Input: part model. Units: mm. Frame: model coordinates. Face numbers are marked on the shaded views. A direction names the side the tool comes from. Coordinates: 2 decimals unless noted, no trailing zeros. Loops run counter-clockwise (first coordinate to the right, second up) from the corner with the lowest first, then second, coordinate; pieces in that order, holes last. Notation, with made-up numbers: (29, 38.5) -> (67, 38.5) arc R33 ccw to (67, 76.5) -> close; hole circle Ø5 at (-6, 40). An arc over 180 degrees is marked (long way). Answer as a JSON object with one key per item and string values.
Autodesk Inventor part; units mm, degrees
ref_plane "YZ Plane" through (0, 0, 0) normal (1, 0, 0) x (0, 1, 0)
ref_plane "XZ Plane" through (0, 0, 0) normal (0, 1, 0) x (-1, 0, 0)
ref_plane "XY Plane" through (0, 0, 0) normal (0, 0, 1) x (1, 0, 0)
sketch "Sketch15" plane through (0, 0, 0) normal (0, 0, 1) x (1, 0, 0)
  line L0 (0, 0) -> (0, 6.6558) construction
  line L1 (0, 0) -> (6.875, 3.9688) construction
  line L2 (6.875, 3.9688) -> (6.875, -3.9688)
  line L3 (6.875, -3.9688) -> (0, 0) construction
  line L4 (6.875, 3.9688) -> (9.3458, 3.9688)
  line L5 (9.3458, 3.9688) -> (9.3458, 3.6433)
  line L6 (9.3458, 3.6433) -> (12.805, 3.6433)
  line L7 (12.805, 3.6433) -> (12.805, 3.9688)
  line L8 (12.805, 3.9688) -> (15.875, 3.9688)
  line L9 (15.875, 3.9688) -> (15.875, 2.3939)
  line L10 (15.875, 2.3939) -> (14.2875, 2.3939)
  line L11 (14.2875, 2.3939) -> (14.2875, -3.9688)
  line L12 (14.2875, -3.9688) -> (12.805, -3.9688)
  line L13 (12.805, -3.9688) -> (12.805, -3.6433)
  line L14 (12.805, -3.6433) -> (9.3458, -3.6433)
  line L15 (9.3458, -3.6433) -> (9.3458, -3.9688)
  line L16 (9.3458, -3.9688) -> (6.875, -3.9688)
  dimension "FlangeOD" = 31.75
  dimension "FlangeThickness" = 1.5748
  dimension "BearingID" = 13.75
  dimension "BearingOD" = 28.575
  dimension "d177" = 7.2866
  dimension "BearingThickness" = 7.9375
  dimension "d179" = 2.4708
  dimension "d180" = 1.4825
  dimension "d181" = 7.4125
revolve "Revolution1" add sketch "Sketch15" angle 360 about axis through (0, 0, 0) along (0, 1, 0)
sketch "Sketch17" plane through (0, 3.9687, 0) normal (0, 1, 0) x (1, 0, 0)
  circle A0 centre (0, 0) radius 6.875
  line L0 (-7.9386, 0) -> (-3.9693, 6.875)
  line L1 (-3.9693, 6.875) -> (3.9693, 6.875)
  line L2 (3.9693, 6.875) -> (7.9386, 0)
  line L3 (7.9386, 0) -> (3.9693, -6.875)
  line L4 (3.9693, -6.875) -> (-3.9693, -6.875)
  line L5 (-3.9693, -6.875) -> (-7.9386, 0)
  point P0 (0, 0)
extrude "Hex" [suppressed]
sketch "Sketch16" plane through (0, 3.6433, 0) normal (0, 1, 0) x (1, 0, 0)
  circle A0 centre (0, 0) radius 9.3458
  circle A1 centre (0, 0) radius 12.805
extrude "Shielded" add sketch "Sketch16" along normal blind 0.127
mirror "Shielded Mirror" about plane through (0, 0, 0) normal (0, 1, 0) of "Shielded"
sketch "Sketch18" plane through (0, 3.6433, 0) normal (0, 1, 0) x (1, 0, 0)
  circle A0 centre (0, 0) radius 2.6458
  circle A1 centre (0, 0) radius 4.1275
extrude "Sealed" [suppressed]
mirror "Sealed Mirror" [suppressed]
equation "\"pi\" = 3.141593"
properties part number "217-4006" material "Steel"
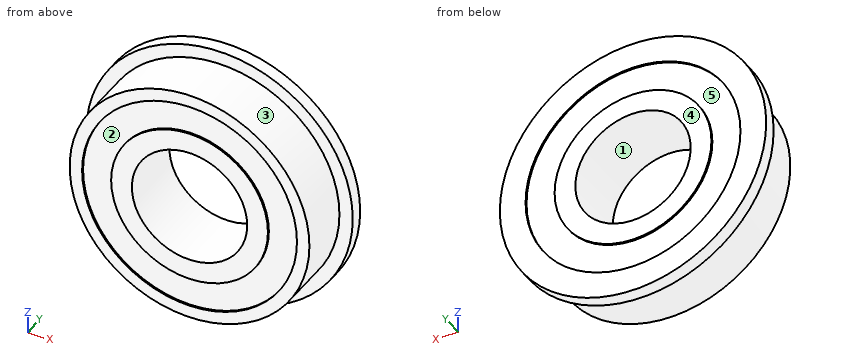
1. Line query: line 1 along X through (y, z) = (3.9, 0) (3 decimals); line 2 along X through (y, z) = (-3.85, 0) (1 decimal); line 3 along Z through (x, y) = (0, -1.25) (1 decimal). Output: solid intervals per line, ascending.
Reply:
{"line 1": "x = -15.875 to -12.805, -9.346 to -6.875, 6.875 to 9.346, 12.805 to 15.875", "line 2": "x = -14.3 to -12.8, -9.3 to -6.9, 6.9 to 9.3, 12.8 to 14.3", "line 3": "z = -14.3 to -6.9, 6.9 to 14.3"}
2. Access query for the marked faces 1 and 2. Directions: +Z, -Z, +X, -X, +Y, -Y. A direction counts if a zero-diameter tool reaches every point of the face in a straight line with its end or side. Return the directions, or none.
Reply:
{"face 1": "+Y, -Y", "face 2": "-Y"}
3. Section query D-D (z = -8.5). Return loops of the section in (x, y), plus the area to 3 significant figures.
Reply:
{"outline": "(-13.41, 2.39) -> (-11.48, 2.39) -> (-11.48, -3.97) -> (-9.58, -3.97) -> (-9.58, -3.77) -> (-3.89, -3.77) -> (-3.89, -3.97) -> (3.89, -3.97) -> (3.89, -3.77) -> (9.58, -3.77) -> (9.58, -3.97) -> (11.48, -3.97) -> (11.48, 2.39) -> (13.41, 2.39) -> (13.41, 3.97) -> (9.58, 3.97) -> (9.58, 3.77) -> (3.89, 3.77) -> (3.89, 3.97) -> (-3.89, 3.97) -> (-3.89, 3.77) -> (-9.58, 3.77) -> (-9.58, 3.97) -> (-13.41, 3.97) -> close", "area": "184 mm2"}
4. Mould query, pull axis Z, two halves, no side actions, for the marked faces 3, 4 and 5. Classes: pulls with the +Z half, pulls with the -Z half, needs draft (parallel to the pull), parting line crosses it, or undercut.
Reply:
{"face 3": "parting line crosses it", "face 4": "needs draft", "face 5": "undercut"}
5. Section query B-B (z = 5.5). Return loops of the section in (x, y) (3 decimals), plus the area to 3 significant figures.
Reply:
{"outline": "(-14.892, 2.394) -> (-13.186, 2.394) -> (-13.186, -3.969) -> (-11.564, -3.969) -> (-11.564, -3.77) -> (-7.556, -3.77) -> (-7.556, -3.969) -> (-4.125, -3.969) -> (-4.125, 3.969) -> (-7.556, 3.969) -> (-7.556, 3.77) -> (-11.564, 3.77) -> (-11.564, 3.969) -> (-14.892, 3.969) -> close; (4.125, -3.969) -> (7.556, -3.969) -> (7.556, -3.77) -> (11.564, -3.77) -> (11.564, -3.969) -> (13.186, -3.969) -> (13.186, 2.394) -> (14.892, 2.394) -> (14.892, 3.969) -> (11.564, 3.969) -> (11.564, 3.77) -> (7.556, 3.77) -> (7.556, 3.969) -> (4.125, 3.969) -> close", "area": "146 mm2"}
6. Pin query (flat end, axial travel): P1, Ø1, axis at x = -4.5, y = 2, coming from the -Z side; P2, Ø1, axis at x = 6, y = 1.5, coming from the +Z side; P3, Ø1.5, axis at x = -10, y = -2.5, coming from the -Z side. Return the tip coordinate at first contact, or that it passes through.
Reply:
{"P1": "stops at z = -15.31", "P2": "stops at z = 13.19", "P3": "stops at z = -10.89"}
